Autodesk Inventor part; units mm, degrees
ref_plane "YZ Plane" through (0, 0, 0) normal (1, 0, 0) x (0, 1, 0)
ref_plane "XZ Plane" through (0, 0, 0) normal (0, 1, 0) x (-1, 0, 0)
ref_plane "XY Plane" through (0, 0, 0) normal (0, 0, 1) x (1, 0, 0)
sketch "Sketch1" plane through (0, 0, 0) normal (0, 0, 1) x (1, 0, 0)
  line L0 (0, 0) -> (-6.35, 6.35)
  line L1 (-6.35, 6.35) -> (-103.1386, 3.175)
  line L2 (0, 0) -> (-6.35, -6.35)
  line L3 (-6.35, -6.35) -> (-103.1386, -3.175)
  arc A0 (-103.1386, 3.175) -> (-103.1386, -3.175) centre (0, 0) ccw
  line L4 (0, 0) -> (24.3963, 0) construction
  dimension "d0" = 103.1875
  dimension "d1" = 6.35
  dimension "d2" = 6.35
  dimension "d8" = 135
extrude "Extrusion1" add sketch "Sketch1" along normal blind 6.35
fillet "Fillet1" radius 3.81 2 edges at (-54.7443, -4.7625, 6.35) (-54.7443, 4.7625, 6.35)
properties part number "Lift_Support"
Read the model definition and answer for the solid it produces. Units are mm, in the model's axes. A direction names the side the tool comes from. Round coordinates to 2 decimals unless told otherwise and drop trailing zeros. Loops run counter-clockwise (first coordinate to the right, second up) from the corner with the lowest first, then second, coordinate; pieces in that order, holes last. Notation, with made-up numbers: (17, 87.5) -> (60, 87.5) arc R25 cw to (60, 118.5) -> close; hole circle Ø9 at (-39.5, -28). An arc over 180 degrees is marked (long way). One line per item, written item: value.
1) A cutting plane is placed at A-A (z = 1.25). Determine the outline of the cut face in (x, y) (3 decimals).
Answer list:
outline: (-103.139, -3.175) -> (-6.35, -6.35) -> (0, 0) -> (-6.35, 6.35) -> (-103.139, 3.175) arc R103.187 ccw to start
2) For faces 1 (the face through (-41, 0, 0)), 2 (the face through (-52.3, -3.7, 5.26)), 3 (the face through (-52.3, 3.76, 5.2)), determine the directions among +Z, -Z, +X, -X, +Y, -Y from which every point of the face is accessible in a straight line to the end or side of a thin tool.
Answer list:
face 1: -Z, +X, -X, +Y, -Y
face 2: +Z, -X, -Y
face 3: +Z, -X, +Y
3) Flat-ended cylindrical pins translate along their axes: P1, Ø3, axis at x = -41, z = 1, coming from the -Y side; P2, Ø2, axis at x = -22, z = 5, coming from the +Y side. Find the tip coordinate at first contact, or state that the pin passes through.
Answer list:
P1: stops at y = -5.26
P2: stops at y = 5.55
4) Consider L1, parallel to Z at x = -42.5, y = -1.5; L2, parallel to Y at x = -14.5, z = 5.25; L3, parallel to Y at x = -40, z = 1.5. Determine where each line is inside the solid, lowest interval first. Write a range as [from, to].
Answer list:
L1: z = [0, 6.35]
L2: y = [-4.95, 4.95]
L3: y = [-5.25, 5.25]
